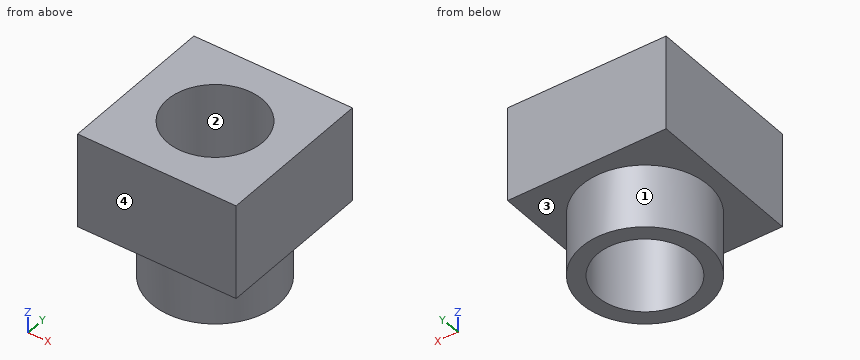
from build123d import *

# Parameters (mm, degrees)
F0_W     = 127
F0_H     = 127
F1_DEPTH = 38.1
F2_R     = 50.8
F3_DEPTH = 50.8
F4_R     = 38.1
F5_DEPTH = 127.001


with BuildPart() as f1:
    # F0 (on Top) → F1 (new body, symmetric)
    with BuildSketch(Plane.XY):
        Rectangle(F0_W, F0_H)
    extrude(amount=F1_DEPTH, both=True)

    # F2 (on face) → F3 (join)
    with BuildSketch(Plane(origin=(0, 0, -38.1), x_dir=(1, 0, 0), z_dir=(0, 0, -1))):
        Circle(F2_R)
    extrude(amount=F3_DEPTH)

    # F4 (on face) → F5 (cut, through all)
    with BuildSketch(Plane(origin=(0, 0, -88.9), x_dir=(1, 0, 0), z_dir=(0, 0, -1))):
        Circle(F4_R)
    extrude(amount=-F5_DEPTH, mode=Mode.SUBTRACT)


solid = f1.part
Can you work these out from the model? Positions are in its coordinate system, mm. Face numbers are marked on the shaded views. Coordinates: 2 decimals unless noted, no trailing zeros. Write each loop counter-clockwise with the first axis right and the second up, starting at its lowest first coordinate (ties: lowest second). Pieces come first, ordered by that corner, then holes. Notation, with made-up numbers: (44.25, 78) -> (59.25, 78) arc R18 ccw to (59.25, 110) -> close; hole circle Ø11 at (30.5, 5.5). An arc over 180 degrees is marked (long way). Answer as CSV lines item,"result".
1) If we section it at C-C on z = -8.5: Please give me the cut outline in (x, y).
Check result:
outline,"(-63.5, -63.5) -> (63.5, -63.5) -> (63.5, 63.5) -> (-63.5, 63.5) -> close; hole circle Ø76.2 at (0, 0)"
2) If I drill on line 1 (Y direction, x = 0, z = -47); line 2 (X direction, y = 0, z = 3), over which ranges is the centre line in solid material (lowest first)? Write a range as from..to.
Check result:
line 1,"-50.8..-38.1, 38.1..50.8"
line 2,"-63.5..-38.1, 38.1..63.5"
3) Will these pins go through, and if not, where does the flat tip stop? P1, Ø3, axis at x = -45.5, y = 49, coming from the -Z side; P2, Ø4, axis at y = 29.5, z = -40.5, coming from the +X side.
Check result:
P1,"z = -38.1"
P2,"x = 42.71"
4) If we section it at D-D on x = 44.5: Please give me the cut outline in (y, z), then the cut area to 3 significant figures.
Check result:
outline,"(-63.5, -38.1) -> (-24.5, -38.1) -> (-24.5, -88.9) -> (24.5, -88.9) -> (24.5, -38.1) -> (63.5, -38.1) -> (63.5, 38.1) -> (-63.5, 38.1) -> close"
area,"12,200 mm²"
5) If we mould it in two halves opening along Y, with no side actions, what happens to the marked faces 1, 2, 3 and 4? For each: +Y half, -Y half, draft (parallel to the pull), parting line (faces both ways), or undercut.
Check result:
face 1,"parting line"
face 2,"undercut"
face 3,"draft"
face 4,"-Y half"
6) If we section it at A-A on y = 0: Please give me the cut outline in (x, z), then the cut area to 3 significant figures.
Check result:
outline,"(-63.5, -38.1) -> (-50.8, -38.1) -> (-50.8, -88.9) -> (-38.1, -88.9) -> (-38.1, 38.1) -> (-63.5, 38.1) -> close; (38.1, -88.9) -> (50.8, -88.9) -> (50.8, -38.1) -> (63.5, -38.1) -> (63.5, 38.1) -> (38.1, 38.1) -> close"
area,"5,160 mm²"
